from build123d import *

# Parameters (mm, degrees)
SKETCH_2_R          = 12
SKETCH_2_R_2        = 5.75
CUT_EXTRUDE_1_DEPTH = 1.15
SKETCH_3_R          = 12
SKETCH_3_R_2        = 5.75
CUT_EXTRUDE_2_DEPTH = 1.15


with BuildPart() as part:
    # ｽｹｯﾁ1 → 回転1 (revolve)
    with BuildSketch(Plane.XY):
        Polygon((0, 0), (0, 5.5), (0.5, 6), (141.5, 6), (142, 5.5), (142, 0), align=None)
    revolve(axis=Axis((142, 0, 0), (-1, 0, 0)))

    # ｽｹｯﾁ2 → ｶｯﾄ - 押し出し1 (cut)
    with BuildSketch(Plane(origin=(5, 0, 0), x_dir=(0, 0, -1), z_dir=(1, 0, 0))):
        Circle(SKETCH_2_R)
        Circle(SKETCH_2_R_2, mode=Mode.SUBTRACT)
    extrude(amount=-CUT_EXTRUDE_1_DEPTH, mode=Mode.SUBTRACT)

    # ｽｹｯﾁ3 → ｶｯﾄ - 押し出し2 (cut)
    with BuildSketch(Plane(origin=(137, 0, 0), x_dir=(0, 0, -1), z_dir=(1, 0, 0))):
        Circle(SKETCH_3_R)
        Circle(SKETCH_3_R_2, mode=Mode.SUBTRACT)
    extrude(amount=CUT_EXTRUDE_2_DEPTH, mode=Mode.SUBTRACT)


solid = part.part
Here's how the part is built. I have some questions about the finished solid (model axes, mm). A direction names the side the tool comes from. Coordinates: 2 decimals unless noted, no trailing zeros. Loops run counter-clockwise (first coordinate to the right, second up) from the corner with the lowest first, then second, coordinate; pieces in that order, holes last.
1. If we mould it in two halves opening along X, with no side actions, what happens to faces 1 (the flat face through (0, 0, 0)), 2 (the cylindrical face through (137.57, 5.7, 0.75)), 3 (the cylindrical face through (140, -6, 0))? For each: pulls with the +X half, pulls with the -X half, needs draft (parallel to the pull), parting line crosses it, or undercut.
2. I need wall thicknesses on L1, parallel to Y at x = 65.5, z = 0.5; L2, parallel to Z at x = 82, y = -0.25; L3, parallel to Z at x = 20, y = 1.5. Which ranges of each line are inside material? Lowest first, please.
3. Imagine slicing it at A-A, the plane x = 22. Please give me the cut outline in (y, z), and give its area (3 significant figures).
4. For faces 4 (the cylindrical face through (2, -6, 0)), 5 (the cylindrical face through (4.43, 5.7, 0.75)), which set-ups out of +Z, -Z, +X, -X, +Y, -Y let a thin tool reach every point of the face, with its end or its side?
Taken from the geometry:
1. face 1: pulls with the -X half
1. face 2: undercut
1. face 3: needs draft
2. L1: y = -5.98 to 5.98
2. L2: z = -5.99 to 5.99
2. L3: z = -5.81 to 5.81
3. outline: circle Ø12 at (0, 0)
3. area: 113 mm2
4. face 4: +X, -X
4. face 5: none
